Can you work these out from the drawing? Everything is in mm from the part's minimum corner. Coordinates: 2 decimals unless noted, no trailing zeros. Order: outer loops, then holes, each group sorted by start corner. A loop starts at its lowest first (then second) coordinate and runs counter-clockwise, first axis right, second up. Notation, with made-up numbers: M 8,22 L 21,22 A6 ccw 21,29 Z; hole C 44,59.5 d5. An arc over 180 degrees is marked long. Answer as a JSON object with one key per item and string values.
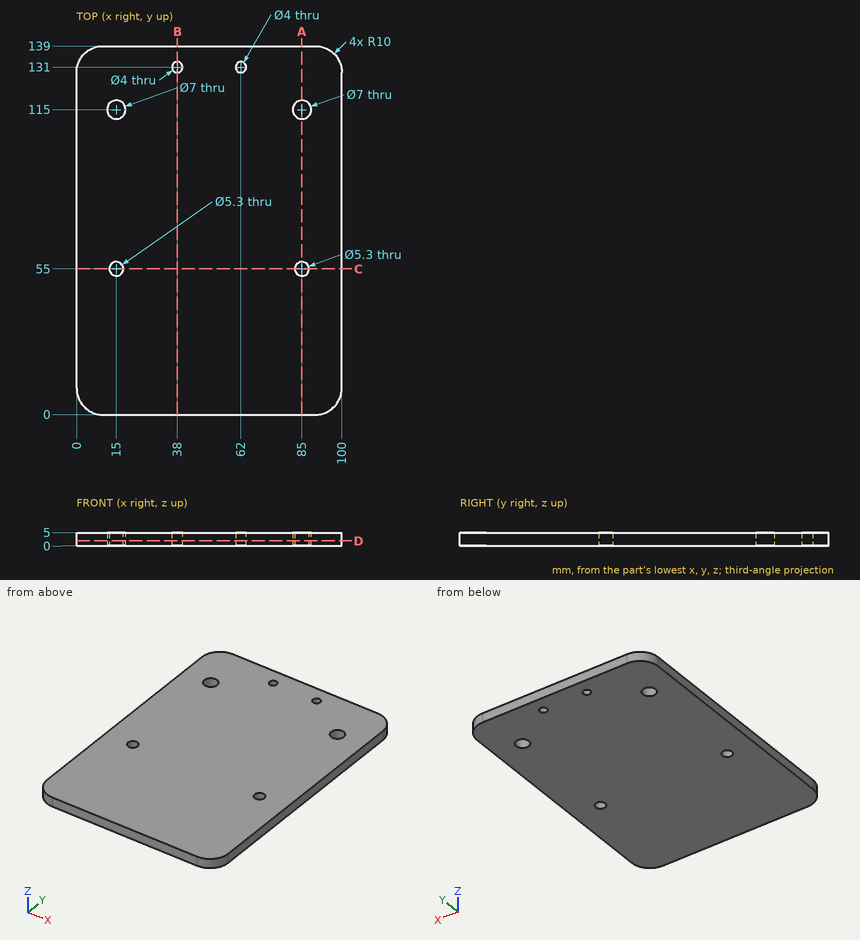
Item 1: I'm going to push a flat-ended pin straight in: pin 1 (11 mm diameter, centred on x = 15, y = 115, fed in from -Z). Where does the tip first touch, or does it pass through?
Answers follow:
{"pin 1": "stops at z = 0"}
Item 2: Please list where these lines run through material, in increasing order: line 1 (Y direction, x = 15, z = 2.25); line 2 (X direction, y = 117, z = 3.1); line 3 (X direction, y = 131, z = 2.4).
Answers follow:
{"line 1": "y = 0 to 52.35, 57.65 to 111.5, 118.5 to 139", "line 2": "x = 0 to 12.13, 17.87 to 82.13, 87.87 to 100", "line 3": "x = 0.2 to 36, 40 to 60, 64 to 99.8"}
Item 3: I want a section at D-D, the plane z = 1.9. Write out the boundary of the cut face in (x, y), plus the area to 3 significant figures.
Answers follow:
{"outline": "M 0,10 A10 ccw 10,0 L 90,0 A10 ccw 100,10 L 100,129 A10 ccw 90,139 L 10,139 A10 ccw 0,129 Z; hole C 15,115 d7; hole C 15,55 d5.3; hole C 38,131 d4; hole C 62,131 d4; hole C 85,115 d7; hole C 85,55 d5.3", "area": "13,700 mm^2"}
Item 4: I want a section at A-A, the plane x = 85. Write out the boundary of the cut face in (y, z), plus the area to 4 significant figures.
Answers follow:
{"outline": "M 0,0 L 52.35,0 L 52.35,5 L 0,5 Z; M 57.65,0 L 111.5,0 L 111.5,5 L 57.65,5 Z; M 118.5,0 L 139,0 L 139,5 L 118.5,5 Z", "area": "633.5 mm^2"}
Item 5: I want a section at C-C, the plane y = 55. Write out the boundary of the cut face in (x, z), plus the area to 3 significant figures.
Answers follow:
{"outline": "M 0,0 L 12.35,0 L 12.35,5 L 0,5 Z; M 17.65,0 L 82.35,0 L 82.35,5 L 17.65,5 Z; M 87.65,0 L 100,0 L 100,5 L 87.65,5 Z", "area": "447 mm^2"}
Item 6: I want a section at B-B, the plane x = 38. Write out the boundary of the cut face in (y, z).
Answers follow:
{"outline": "M 0,0 L 129,0 L 129,5 L 0,5 Z; M 133,0 L 139,0 L 139,5 L 133,5 Z"}
